The listing builds one solid part. Answer for the finished solid, in the listing's coordinates (mm). Face numbers are marked on the shaded views. A direction names the side the tool comes from. Give positions to 0.01 mm unless a question says otherwise; leave off trailing zeros. Order: outer loops, then holes, each group sorted by start corner. A loop starts at its lowest first (then second) coordinate and runs counter-clockwise, first axis right, second up. Notation, with made-up numbers: (-22, 78) - (33, 78) arc R32 cw to (33, 107) - close; hole circle Ø11 at (23.25, -29.75). An arc over 180 degrees is marked (long way). Answer as a JSON object with one key per item and string values. Group by question number.
Q1. For the marked faces 1, 2 and 3, determine the directions among +Z, -Z, +X, -X, +Y, -Y from which every point of the face is accessible in a straight line to the end or side of a thin tool.
Q2. A cutting plane is placed at C-C, the plane x = 0. Give the vertices of the cut face in (y, z).
Q3. A cutting plane is placed at A-A, the plane y = 0. Give the vertices of the cut face in (x, z).
Q4. A cutting plane is placed at B-B, the plane z = 0. Give the vertices of the cut face in (x, y), and give its area (3 significant figures).
Q5. Given pin 1 (1 mm diameter, centred on x = 3.5, z = 1, fed in from -Y); pin 2 (5 mm diameter, centred on x = 1.5, y = 41, fed in from +Z), each flat-ended and moving along its own axis, determine where each tip first touches the part or whether it passes through.
Q6. Consider line 1 (Z direction, x = 2.25, y = 0); line 2 (Y direction, x = 1, z = 0.5); line 3 (Y direction, x = 4, z = -3.25). Determine where each line is inside the solid, lowest interval first.
from build123d import *

# Parameters (mm, degrees)
F0_W     = 64
F0_H     = 10
F0_R     = 2.5
F1_DEPTH = 5
F3_START = 9
F2_R     = 3
F3_DEPTH = 43
F4_START = -10
F4_DEPTH = 42


with BuildPart() as f1:
    # F0 (on Right) → F1 (new body, symmetric)
    with BuildSketch(Plane.YZ):
        Rectangle(F0_W, F0_H)
        Circle(F0_R, mode=Mode.SUBTRACT)
    extrude(amount=F1_DEPTH, both=True)

    # F2 (on Front) → F3 (join)
    with BuildSketch(Plane.XZ.offset(F3_START)):
        Circle(F2_R)
    extrude(amount=F3_DEPTH)

    # F2 (on Front) → F4 (join)
    with BuildSketch(Plane.XZ.offset(F4_START)):
        Circle(F2_R)
    extrude(amount=-F4_DEPTH)


solid = f1.part
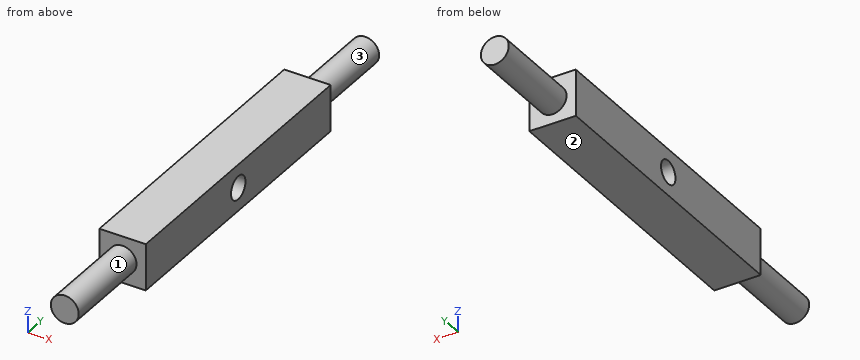
Reply:
{
 "1": {"face 1": "-Y", "face 2": "-Z, +X, -X, +Y, -Y", "face 3": "+Y"},
 "2": {"outline": "(-52, -3) - (-32, -3) - (-32, -5) - (32, -5) - (32, -3) - (52, -3) - (52, 3) - (32, 3) - (32, 5) - (-32, 5) - (-32, 3) - (-52, 3) - close; hole circle Ø5 at (0, 0)"},
 "3": {"outline": "(-5, -5) - (5, -5) - (5, -2.5) - (-5, -2.5) - close; (-5, 2.5) - (5, 2.5) - (5, 5) - (-5, 5) - close"},
 "4": {"outline": "(-5, -32) - (-3, -32) - (-3, -52) - (3, -52) - (3, -32) - (5, -32) - (5, -2.5) - (-5, -2.5) - close; (-5, 2.5) - (5, 2.5) - (5, 32) - (3, 32) - (3, 52) - (-3, 52) - (-3, 32) - (-5, 32) - close", "area": "830 mm^2"},
 "5": {"pin 1": "stops at y = -32", "pin 2": "stops at z = 3"},
 "6": {"line 1": "z = -5 to -2.5, 2.5 to 5", "line 2": "y = -52 to -2.45, 2.45 to 52", "line 3": "y = -32 to 32"}
}
